```python
from build123d import *

# Parameters (mm, degrees)
F0_R     = 0.762
F0_R_2   = 14.3129
F1_DEPTH = 3.175
F2_R     = 2.54


with BuildPart() as f1:
    # F0 (on Top) → F1 (new body)
    with BuildSketch(Plane.XY):
        with BuildLine():
            ThreePointArc((37.814818885, -4.6528993857), (16.2183640692, 8.713670097), (16.9939270688, 34.1000944688))
            ThreePointArc((16.9939270688, 34.1000944688), (1.1909176957, 38.0813827879), (-14.8299813197, 35.0953223957))
            ThreePointArc((-14.8299813197, 35.0953223957), (-15.6508840085, 9.7188762367), (-38.0323831061, -2.2688841474))
            ThreePointArc((-38.0323831061, -2.2688841474), (-33.5888120947, -17.9833729335), (-22.9742885145, -30.3939478721))
            ThreePointArc((-22.9742885145, -30.3939478721), (-0.5866848831, -18.4058352173), (20.9920077442, -31.7953709031))
            ThreePointArc((20.9920077442, -31.7953709031), (32.3842423806, -20.0716428185), (37.814818885, -4.6528993857))
        make_face()
        with BuildLine():
            ThreePointArc((-22.6742041591, -21.077906737), (-30.5143778905, -16.2115761649), (-30.2921493088, -6.9866039788))
            Line((-30.2921493088, -6.9866039788), (-22.6742041591, -21.077906737))
        make_face(mode=Mode.SUBTRACT)
        with Locations((-9.7768361415, -15.7612173143)):
            Circle(F0_R, mode=Mode.SUBTRACT)
        with BuildLine():
            ThreePointArc((-22.077246757, -2.5455187134), (-14.2471455868, -7.4172946457), (-14.4593016073, -16.6368214716))
            Line((-14.4593016073, -16.6368214716), (-22.077246757, -2.5455187134))
        make_face(mode=Mode.SUBTRACT)
        with Locations((8.761196518, -16.3475971243)):
            Circle(F0_R, mode=Mode.SUBTRACT)
        with BuildLine():
            ThreePointArc((12.5619529023, -18.1867123268), (12.756507598, -9.1097250706), (20.6001486004, -4.5373247159))
            Line((20.6001486004, -4.5373247159), (12.5619529023, -18.1867123268))
        make_face(mode=Mode.SUBTRACT)
        with Locations((18.5380326595, -0.58637981)):
            Circle(F0_R, mode=Mode.SUBTRACT)
        with BuildLine():
            Line((20.8666791326, -23.0774090058), (28.9048748307, -9.4280213948))
            ThreePointArc((28.9048748307, -9.4280213948), (28.7016006579, -18.4998737054), (20.8666791326, -23.0774090058))
        make_face(mode=Mode.SUBTRACT)
        with Locations((-18.5380326595, 0.58637981)):
            Circle(F0_R, mode=Mode.SUBTRACT)
        with Locations((-8.761196518, 16.3475971243)):
            Circle(F0_R, mode=Mode.SUBTRACT)
        Circle(F0_R_2, mode=Mode.SUBTRACT)
        with BuildLine():
            ThreePointArc((8.554840384, 20.4151336434), (0.3927024044, 16.1488375122), (-7.4634526605, 20.9553546163))
            Line((-7.4634526605, 20.9553546163), (8.554840384, 20.4151336434))
        make_face(mode=Mode.SUBTRACT)
        with Locations((9.7768361415, 15.7612173143)):
            Circle(F0_R, mode=Mode.SUBTRACT)
        with BuildLine():
            Line((8.86910012, 29.7333659897), (-7.1491929245, 30.2735869625))
            ThreePointArc((-7.1491929245, 30.2735869625), (1.0136418787, 34.5605448721), (8.86910012, 29.7333659897))
        make_face(mode=Mode.SUBTRACT)
    extrude(amount=F1_DEPTH)

    # F2
    f2_edges = [f1.edges().sort_by_distance(p)[0] for p in [
        (-0.586685, -18.405835, 3.175),
        (1.190918, 38.081383, 3.175),
        (-15.650884, 9.718876, 3.175),
        (-33.588812, -17.983373, 3.175),
        (16.218364, 8.71367, 3.175),
        (32.384242, -20.071643, 3.175),
    ]]
    fillet(f2_edges, radius=F2_R)


solid = f1.part
```
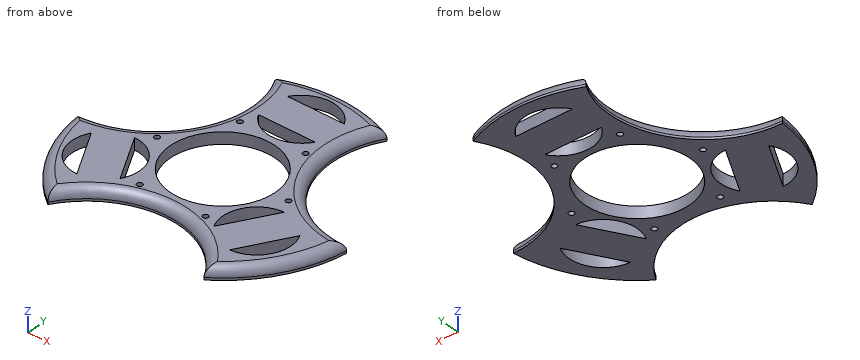
Could you check a few things on this model? Use its own coordinates, in mm. Give positions to 0.01 mm unless a question says otherwise; leave off trailing zeros. Use one line per item in the form item = value.
1. I want a section at A-A (z = 2.45). Give the number of separate pieces and of enclosed holes in the cut face, and give its area (3 significant figures).
Response values:
separate_pieces = 1
enclosed_holes = 13
area = 1,590 mm²
2. I need wall thicknesses on probe 1 along Y at (x, z) = (4.5, 0.5); probe 2 along Y at (x, z) = (21, 2.5); probe 3 along Y at (x, z) = (-28, 1.55). Which ranges of each line are inside material? Lowest first, please.
Response values:
probe_1 = -19.09 to -13.59, 13.59 to 16.95, 20.55 to 29.88, 33.76 to 37.83
probe_2 = -30.17 to -23.07, -22.85 to 1.3
probe_3 = -25.59 to -19.16, -11.23 to -0.73
3. I'm going to push flat-ended pins straight in: pin 1 Ø2 at (x, y) = (18.5, 0.5) entering from -Z; pin 2 Ø1.5 at (x, z) = (18, 3) entering from -Y; pin 3 Ø1 at (x, z) = (-18.5, 2) entering from +Y. Where does each tip first touch, or does it pass through?
Response values:
pin_1 = 0
pin_2 = -26.82
pin_3 = 6.06
